Check sheet for the modelled part. Datum: model origin and axes. Units: mm. Round coordinates to 2 decimals unless told otherwise and drop trailing zeros. Order: outer loops, then holes, each group sorted by start corner. A loop starts at its lowest first (then second) coordinate and runs counter-clockwise, first axis right, second up.
Autodesk Inventor part; units mm, degrees
ref_plane "YZ Plane" through (0, 0, 0) normal (1, 0, 0) x (0, 1, 0)
ref_plane "XZ Plane" through (0, 0, 0) normal (0, 1, 0) x (-1, 0, 0)
ref_plane "XY Plane" through (0, 0, 0) normal (0, 0, 1) x (1, 0, 0)
sketch "Sketch1" plane through (0, 0, 0) normal (0, 0, 1) x (1, 0, 0)
  line L0 (-692.5, -1287.5) -> (692.5, -1287.5)
  line L1 (692.5, -1287.5) -> (692.5, 1287.5)
  line L2 (692.5, 1287.5) -> (-692.5, 1287.5)
  line L3 (-692.5, 1287.5) -> (-692.5, -1287.5)
  line L4 (-692.5, -1287.5) -> (692.5, 1287.5) construction
  line L5 (692.5, -1287.5) -> (-692.5, 1287.5) construction
  line L6 (692.5, -1247.5) -> (652.5, -1247.5)
  line L7 (652.5, -1247.5) -> (652.5, -1287.5)
  line L8 (692.5, 1222.5) -> (652.5, 1222.5)
  line L9 (652.5, 1222.5) -> (652.5, 932.5)
  line L10 (652.5, 932.5) -> (692.5, 932.5)
  line L11 (692.5, 932.5) -> (692.5, 1222.5)
  line L12 (652.5, 1067.5) -> (642.5, 1067.5)
  line L13 (642.5, 1067.5) -> (642.5, 1217.5)
  line L14 (642.5, 1217.5) -> (652.5, 1217.5)
  line L15 (-572.5, -767.5) -> (17.5, -767.5)
  line L16 (17.5, -767.5) -> (17.5, -177.5)
  line L17 (17.5, -177.5) -> (-572.5, -177.5)
  line L18 (-572.5, -177.5) -> (-572.5, -767.5)
  point P0 (0, 0)
  dimension "d154" = 1385
  dimension "d155" = 2575
  dimension "d157" = 40
  dimension "d159" = 290
  dimension "d161" = 40
  dimension "d162" = 2220
  dimension "d163" = 10
  dimension "d164" = 150
  dimension "d165" = 5
  dimension "d166" = 590
  dimension "d167" = 590
  dimension "d168" = 675
  dimension "d169" = 520
extrude "Plate5" add sketch "Sketch1" along normal blind 2 contours L3 L2 L1 L8 L9 L14 L13 L12 L10 L6 L7 L0
fillet "Corner Round1" radius 15 1 edges at (652.5, -1247.5, 1)
properties part number "PNS-0111 floor sheet 2" material "Stainless Steel"
Item 1: Sectioned sample at D-D (y = 957). Record the cut outline in (x, z), and give its area (3 significant figures).
Answer:
outline: (-692.5, 0) - (652.5, 0) - (652.5, 2) - (-692.5, 2) - close
area: 2,690 mm2
Item 2: Scan lines: line 1 along Y through (x, z) = (-189, 0.5); line 2 along X through (y, z) = (-407, 1.05); line 3 along X through (y, z) = (1138.5, 0.2). Record each from-to range of solid material in increasing order.
Answer:
line 1: y = -1287.5 to -767.5, -177.5 to 1287.5
line 2: x = -692.5 to -572.5, 17.5 to 692.5
line 3: x = -692.5 to 642.5
Item 3: Sectioned sample at A-A (z = 1). Record the cut outline in (x, y), and give its area (3 significant figures).
Answer:
outline: (-692.5, -1287.5) - (652.5, -1287.5) - (652.5, -1262.5) arc R15 cw to (667.5, -1247.5) - (692.5, -1247.5) - (692.5, 932.5) - (652.5, 932.5) - (652.5, 1067.5) - (642.5, 1067.5) - (642.5, 1217.5) - (652.5, 1217.5) - (652.5, 1222.5) - (692.5, 1222.5) - (692.5, 1287.5) - (-692.5, 1287.5) - close; hole (-572.5, -767.5) - (17.5, -767.5) - (17.5, -177.5) - (-572.5, -177.5) - close
area: 3,200,000 mm2
Item 4: Sectioned sample at C-C (x = -17). Record the cut outline in (y, z).
Answer:
outline: (-1287.5, 0) - (-767.5, 0) - (-767.5, 2) - (-1287.5, 2) - close; (-177.5, 0) - (1287.5, 0) - (1287.5, 2) - (-177.5, 2) - close
Item 5: Sectioned sample at B-B (y = -525.5). Record the cut outline in (x, z).
Answer:
outline: (-692.5, 0) - (-572.5, 0) - (-572.5, 2) - (-692.5, 2) - close; (17.5, 0) - (692.5, 0) - (692.5, 2) - (17.5, 2) - close
Item 6: Go/stop test with flat-tipped pins: P1, Ø0.6, axis at y = 1220, z = 1.5, coming from the +X side; P2, Ø0.6, axis at x = 670, z = 1, coming from the -Y side. Record where each tip stops, or that it passes through.
Answer:
P1: stops at x = 652.5
P2: stops at y = -1247.5
